```python
from build123d import *

# Parameters (mm, degrees)
SKETCH1_R           = 2.125
BOSS_EXTRUDE1_DEPTH = 19.05
FILLET1_R           = 6.35
FILLET2_R           = 6.35
SKETCH3_W           = 63.5
SKETCH3_H           = 63.5
BOSS_EXTRUDE2_DEPTH = 19.05
FILLET3_R           = 76.2
SKETCH8_R           = 2.125
CUT_EXTRUDE3_DEPTH  = 19.05
SKETCH10_R          = 2
CUT_EXTRUDE7_DEPTH  = 335.208156388


with BuildPart() as part:
    # Sketch1 → Boss-Extrude1 (new body)
    with BuildSketch(Plane.XY):
        with BuildLine():
            Line((0, 0), (0, -76.2))
            ThreePointArc((0, -76.2), (152.4, -108.007732044), (304.8, -76.2))
            Line((304.8, -76.2), (304.8, 0))
            ThreePointArc((304.8, 0), (152.4, -72.254002873), (0, 0))
        make_face()
        with Locations(Location((19.05, -57.207732044, 0), (0, 0, 180))):
            Circle(SKETCH1_R, mode=Mode.SUBTRACT)
        with Locations(Location((285.75, -57.207732044, 0), (0, 0, 180))):
            Circle(SKETCH1_R, mode=Mode.SUBTRACT)
    extrude(amount=BOSS_EXTRUDE1_DEPTH)

    # Fillet1
    fillet1_edges = [part.edges().sort_by_distance(p)[0] for p in [
        (304.8, 0, 9.525),
        (0, 0, 9.525),
    ]]
    fillet(fillet1_edges, radius=FILLET1_R)

    # Fillet2
    fillet2_edges = [part.edges().sort_by_distance(p)[0] for p in [
        (304.8, -76.2, 9.525),
        (0, -76.2, 9.525),
    ]]
    fillet(fillet2_edges, radius=FILLET2_R)

    # Sketch3 → Boss-Extrude2 (add)
    with BuildSketch(Plane.XY.offset(19.05)):
        with Locations((152.4, -104.004002873)):
            Rectangle(SKETCH3_W, SKETCH3_H)
    extrude(amount=-BOSS_EXTRUDE2_DEPTH)

    # Fillet3
    # the kernel refuses this fillet: 76.2 mm, written as the material it adds along each edge
    with BuildSketch(Plane(origin=(184.15, -106.682510638, 19.05), x_dir=(0.9888312847973341, 0.1490392237166227, 0), z_dir=(0, 0, -1))) as fillet3_piece_1:
        with BuildLine():
            CenterArc((55.420290143, 76.033258895), FILLET3_R, 218.356834864, 47.852104701)
            Line((-4.332792635, 28.746801018), (-5.527854291, 27.801071861))
            ThreePointArc((-5.527854291, 27.801071861), (-3.673375196, 14.146264732), (-1.506978878, -0.227135777))
            Line((-1.506978878, -0.227135777), (0.100764164, -1.520665178))
            ThreePointArc((0.100764164, -1.520665178), (25.191040974, -0.690294475), (50.281317784, -1.520665178))
            Line((50.281317784, -1.520665178), (50.382081948, 0))
        make_face()
    extrude(amount=19.05)
    with BuildSketch(Plane(origin=(120.65, -106.682510638, 19.05), x_dir=(0, -1, 0), z_dir=(0, 0, -1))) as fillet3_piece_2:
        with BuildLine():
            CenterArc((66.924268059, 66.133254588), FILLET3_R, 192.362312718, 47.852104701)
            Line((-7.508906383, 49.819378823), (-8.997569872, 49.493101308))
            ThreePointArc((-8.997569872, 49.493101308), (-4.437037964, 24.806808459), (-1.518699114, -0.127))
            Line((-1.518699114, -0.127), (0, -1.524))
            ThreePointArc((0, -1.524), (14.535746118, -1.524), (28.314436719, -1.322665092))
            Line((28.314436719, -1.322665092), (29.071492235, 0))
        make_face()
    extrude(amount=19.05)

    # Sketch8 → Cut-Extrude3 (cut)
    with BuildSketch(Plane(origin=(0, 0, 0), x_dir=(-1, 0, 0), z_dir=(0, 0, -1))):
        with Locations((-171.45, -125.902330937)):
            Circle(SKETCH8_R)
        with Locations((-133.35, -125.902330937)):
            Circle(SKETCH8_R)
    extrude(amount=-CUT_EXTRUDE3_DEPTH, mode=Mode.SUBTRACT)

    # Sketch10 → Cut-Extrude7 (cut, through all)
    with BuildSketch(Plane.XY.offset(19.05)):
        with Locations((133.35, -102.618997603)):
            Circle(SKETCH10_R)
        with Locations((171.45, -102.618997603)):
            Circle(SKETCH10_R)
    extrude(amount=-CUT_EXTRUDE7_DEPTH, mode=Mode.SUBTRACT)


solid = part.part
```
Part model, mm, in its own coordinate system. Round coordinates to 2 decimals unless told otherwise and drop trailing zeros. Write each loop counter-clockwise with the first axis right and the second up, starting at its lowest first coordinate (ties: lowest second). Pieces come first, ordered by that corner, then holes.
Item 1: Cut at B-B, the plane z = 7.5. Give the cut face in (x, y) (3 decimals).
Results:
outline: (0, -72.018) arc R6.35 ccw to (3.875, -77.866) arc R381 ccw to (70.831, -99.174) arc R76.2 cw to (120.65, -135.754) - (184.15, -135.754) arc R76.2 cw to (233.969, -99.174) arc R381 ccw to (300.925, -77.866) arc R6.35 ccw to (304.8, -72.018) - (304.8, -16.683) arc R6.35 ccw to (293.886, -12.268) arc R196.85 cw to (10.914, -12.268) arc R6.35 ccw to (0, -16.683) - close; hole circle Ø4.25 at (19.05, -57.208); hole circle Ø4.25 at (133.35, -125.902); hole circle Ø4 at (133.35, -102.619); hole circle Ø4.25 at (171.45, -125.902); hole circle Ø4 at (171.45, -102.619); hole circle Ø4.25 at (285.75, -57.208)
Item 2: Drop flat-ended pins along their axis: pin 1 Ø8 at (x, z) = (73.5, 2.5) entering from +Y; pin 2 Ø4 at (x, z) = (79, 7) entering from -Y; pin 3 Ø3 at (x, z) = (149, 9) entering from +Y; pin 4 Ø2.5 at (x, y) = (133.35, -125.9) entering from +Z. Give the stop position or say it passes through.
Results:
pin 1: stops at y = -53.95
pin 2: stops at y = -102.16
pin 3: stops at y = -72.19
pin 4: passes through
Item 3: Cut at D-D, the plane x = 102.5. Give the cut face in (y, z).
Results:
outline: (-114.41, 0) - (-65.82, 0) - (-65.82, 19.05) - (-114.41, 19.05) - close
Item 4: Two-plate mould, pull along X, no slides. Class faces 1 (the cylindrical face through (154.61, -72.24, 9.39)), 2 (the flat face through (150, -74, 0)), 3 (the flat face through (304.8, -45, 9)), 4 (the cylindrical face through (36.391, -89.917, 9.392)): +X half, -X half, draft (parallel to the pull), parting line (faces both ways), or undercut.
Results:
face 1: undercut
face 2: draft
face 3: +X half
face 4: -X half
Item 5: Cut at C-C, the plane x = 214. Give the cut face in (y, z).
Results:
outline: (-106.6, 0) - (-62.37, 0) - (-62.37, 19.05) - (-106.6, 19.05) - close
Item 6: Probe L1, parallel to Y at x = 135, z = 12.5; L2, parallel to Y at x = 171.45, z = 12.5; L3, parallel to X at y = -55.5, z = 11.75. List the from-to ranges inside material, lowest first.
Results:
L1: y = -135.75 to -127.24, -124.56 to -103.75, -101.49 to -71.48
L2: y = -135.75 to -128.03, -123.78 to -104.62, -100.62 to -71.33
L3: x = 0 to 17.79, 20.31 to 72.93, 231.87 to 284.49, 287.01 to 304.8
Item 7: Cut at A-A, the plane y = -40. Give the cut face in (x, z).
Results:
outline: (0, 0) - (44.43, 0) - (44.43, 19.05) - (0, 19.05) - close; (260.37, 0) - (304.8, 0) - (304.8, 19.05) - (260.37, 19.05) - close
